Geometry: final body of the model. Coordinates: model frame, mm. A direction names the side the tool comes from. Round coordinates to 2 decimals unless told otherwise and drop trailing zeros. Write each loop counter-clockwise with the first axis right and the second up, starting at its lowest first coordinate (ties: lowest second). Pieces come first, ordered by that corner, then holes. Notation, with made-up numbers: (-35.5, 65) -> (7.5, 65) arc R15 ccw to (7.5, 91) -> close; hole circle Ø6 at (34.25, 50.5). An arc over 180 degrees is marked (long way). Use one line per item in the form item = value. Start each with the question number.
1. Cut plane D-D, the plane x = -69.25. Return the cut outline in (y, z), plus the area to 3 significant figures.
2. Reachability of faces 1 (the face through (-45.97, -344.33, 13.56)), 2 (the face through (-60, -173, 2.5)) from +Z, -Z, +X, -X, +Y, -Y: full face, straight path, thin tool, end or side. Return the list, or none.
3. Cut plane C-C, the plane y = -195. Return the cut outline in (x, z), plus the area to 4 significant figures.
4. Cut plane A-A, the plane z = 13.75. Return the cut outline in (x, y), plus the area to 3 significant figures.
5. Line query: L1, parallel to Z at x = -46.05, y = -20; L2, parallel to X at y = -228, z = 10.75; L3, parallel to Z at x = -63, y = -266.5. Output: solid intervals per line, ascending.
6. Pin query (flat end, axial travel): pin 1 Ø11.5 at (y, z) = (-20, 13.75) entering from +X; pin 2 Ø9 at (y, z) = (-20, 13.75) entering from +X. Return the tip coordinate at first contact, or that it passes through.
7. Draft query along Z for faces 3 (the face through (-74.986, -173, 14)), 4 (the face through (-60, -173, 27.5)), 5 (the face through (-60, -173, 0)), 6 (the face through (-73.718, -24.995, 13.97)). Return one class per face: pulls with the +Z half, pulls with the -Z half, needs draft (parallel to the pull), parting line crosses it, or undercut.
8. Cut plane B-B, the plane y = -20. Return the cut outline in (x, z), plus the area to 4 significant figures.
```python
from build123d import *

# Parameters (mm, degrees)
F0_W        = 30
F0_H        = 27.5
F0_W_2      = 25
F0_H_2      = 22.5
F1_DEPTH    = 350
F3_DEPTH    = 53
F4_T1_DEPTH = 77.5
F5_R        = 5
F6_DEPTH    = 37.8


# Not quite as in the source:
# - a fillet or chamfer that OpenCascade refuses, or shapes differently, is made with other operations: its cross-section is extruded or revolved along the edge and cut away or added
# - a feature names something its author has since deleted; it is built from what else it names


with BuildPart() as f1:
    # F0 (on Front) → F1 (new body)
    with BuildSketch(Plane.XZ):
        with Locations((-59.9858543277, 13.75)):
            Rectangle(F0_W, F0_H)
        with Locations((-59.9858543277, 13.75)):
            Rectangle(F0_W_2, F0_H_2, mode=Mode.SUBTRACT)
    extrude(amount=F1_DEPTH)

    # F2 (on Top) → F3 (cut)
    with BuildSketch(Plane.XY):
        with BuildLine():
            Line((-59.9858543277, -340), (-59.9858543277, -335))
            ThreePointArc((-59.9858543277, -335), (-64.9858543277, -340), (-59.9858543277, -345))
            Line((-59.9858543277, -345), (-59.9858543277, -340))
        make_face()
        with BuildLine():
            ThreePointArc((-54.9858543277, -340), (-56.4503204217, -336.4644660941), (-59.9858543277, -335))
            Line((-59.9858543277, -335), (-59.9858543277, -340))
            Line((-59.9858543277, -340), (-59.9858543277, -345))
            ThreePointArc((-59.9858543277, -345), (-56.4503204217, -343.5355339059), (-54.9858543277, -340))
        make_face()
        with BuildLine():
            Line((-59.9858543277, -45), (-59.9858543277, -35))
            ThreePointArc((-59.9858543277, -35), (-64.9858543277, -40), (-59.9858543277, -45))
        make_face()
        with BuildLine():
            ThreePointArc((-54.9858543277, -40), (-56.4503204217, -36.4644660941), (-59.9858543277, -35))
            Line((-59.9858543277, -35), (-59.9858543277, -45))
            ThreePointArc((-59.9858543277, -45), (-56.4503204217, -43.5355339059), (-54.9858543277, -40))
        make_face()
        with BuildLine():
            Line((-59.9858543277, -15), (-59.9858543277, -5))
            ThreePointArc((-59.9858543277, -5), (-64.9858543277, -10), (-59.9858543277, -15))
        make_face()
        with BuildLine():
            ThreePointArc((-59.9858543277, -15), (-56.4503204217, -13.5355339059), (-54.9858543277, -10))
            ThreePointArc((-54.9858543277, -10), (-56.4503204217, -6.4644660941), (-59.9858543277, -5))
            Line((-59.9858543277, -5), (-59.9858543277, -15))
        make_face()
        with BuildLine():
            Line((-59.9858543277, -315), (-59.9858543277, -305))
            ThreePointArc((-59.9858543277, -305), (-64.9858543277, -310), (-59.9858543277, -315))
        make_face()
        with BuildLine():
            ThreePointArc((-54.9858543277, -310), (-56.4503204217, -306.4644660941), (-59.9858543277, -305))
            Line((-59.9858543277, -305), (-59.9858543277, -315))
            ThreePointArc((-59.9858543277, -315), (-56.4503204217, -313.5355339059), (-54.9858543277, -310))
        make_face()
    extrude(amount=F3_DEPTH, mode=Mode.SUBTRACT)

    # F4: fillet of radius 10 on 4 edges, made by hand

    # F4_s2 → F4_t1 (cut)
    with BuildSketch(Plane.XY.offset(-25)):
        with BuildLine():
            ThreePointArc((-74.9858543277, -10), (-72.0569221395, -2.9289321881), (-64.9858543277, 0))
            Line((-64.9858543277, 0), (-74.9858543277, 0))
            Line((-74.9858543277, 0), (-74.9858543277, -10))
        make_face()
        with BuildLine():
            ThreePointArc((-74.9858543277, -340), (-72.0569221395, -347.0710678119), (-64.9858543277, -350))
            Line((-64.9858543277, -350), (-74.9858543277, -350))
            Line((-74.9858543277, -350), (-74.9858543277, -340))
        make_face()
        with BuildLine():
            ThreePointArc((-54.9858543277, 0), (-47.9147865158, -2.9289321881), (-44.9858543277, -10))
            Line((-44.9858543277, -10), (-44.9858543277, 0))
            Line((-44.9858543277, 0), (-54.9858543277, 0))
        make_face()
        with BuildLine():
            ThreePointArc((-54.9858543277, -350), (-47.9147865158, -347.0710678119), (-44.9858543277, -340))
            Line((-44.9858543277, -340), (-44.9858543277, -350))
            Line((-44.9858543277, -350), (-54.9858543277, -350))
        make_face()
    extrude(amount=F4_T1_DEPTH, mode=Mode.SUBTRACT)

    # F5 (on face) → F6 (cut)
    with BuildSketch(Plane.YZ.offset(-44.9858543277)):
        with Locations((-20, 13.75)):
            Circle(F5_R)
    extrude(amount=-F6_DEPTH, mode=Mode.SUBTRACT)


solid = f1.part
```
Outcome:
q1.outline = (-349.05, 0) -> (-0.95, 0) -> (-0.95, 2.5) -> (-349.05, 2.5) -> close; (-349.05, 25) -> (-0.95, 25) -> (-0.95, 27.5) -> (-349.05, 27.5) -> close
q1.area = 1,740 mm^2
q2.face_1 = +Z, -Z, +X, -Y
q2.face_2 = +Y, -Y
q3.outline = (-74.99, 0) -> (-44.99, 0) -> (-44.99, 27.5) -> (-74.99, 27.5) -> close; hole (-72.49, 2.5) -> (-47.49, 2.5) -> (-47.49, 25) -> (-72.49, 25) -> close
q3.area = 262.5 mm^2
q4.outline = (-74.99, -340) arc R10 ccw to (-72.49, -346.61) -> (-72.49, -25) -> (-74.99, -25) -> close; (-74.99, -15) -> (-72.49, -15) -> (-72.49, -3.39) arc R10 ccw to (-74.99, -10) -> close; (-47.49, -346.61) arc R10 ccw to (-44.99, -340) -> (-44.99, -25) -> (-47.49, -25) -> close; (-47.49, -15) -> (-44.99, -15) -> (-44.99, -10) arc R10 ccw to (-47.49, -3.39) -> close
q4.area = 1,650 mm^2
q5.L1 = 0 to 8.75, 18.75 to 27.5
q5.L2 = -74.99 to -72.49, -47.49 to -44.99
q5.L3 = 0 to 2.5, 25 to 27.5
q6.pin_1 = -44.99
q6.pin_2 = through
q7.face_3 = needs draft
q7.face_4 = pulls with the +Z half
q7.face_5 = pulls with the -Z half
q7.face_6 = undercut
q8.outline = (-74.99, 0) -> (-44.99, 0) -> (-44.99, 8.75) -> (-47.49, 8.75) -> (-47.49, 2.5) -> (-72.49, 2.5) -> (-72.49, 8.75) -> (-74.99, 8.75) -> close; (-74.99, 18.75) -> (-72.49, 18.75) -> (-72.49, 25) -> (-47.49, 25) -> (-47.49, 18.75) -> (-44.99, 18.75) -> (-44.99, 27.5) -> (-74.99, 27.5) -> close
q8.area = 212.5 mm^2
